Check sheet for the modelled part. Datum: model origin and axes. Units: mm. A direction names the side the tool comes from. Round coordinates to 2 decimals unless told otherwise and drop trailing zeros. Loops run counter-clockwise (first coordinate to the right, second up) from the corner with the lowest first, then second, coordinate; pieces in that order, holes last. Notation, with made-up numbers: (-19.5, -19.75) - (-9.5, -19.75) arc R24 cw to (-9.5, 14.25) - close; hole circle Ø6 at (-25, -6.5). An arc over 180 degrees is marked (long way). Answer in a Markdown table with one row per item. Add a question column.
(1) Mould release check, pull along X, two halves, no side actions. Record for faces 1 (the cylindrical face through (-0.385, -11.515, -0.022)), 2 (the flat face through (-42, 19, -2.921)), 3 (the cylindrical face through (-11.012, -49.592, 0.041)): +X half, -X half, draft (parallel to the pull), parting line (faces both ways), or undercut.
(2) Cross-section at D-D on y = 28.5. Enter the section's corners in (x, z), then the cut area to 3 significant figures.
(3) Cross-section at C-C on z = -0.25. Count the separate pieces of the cut face and the enclosed holes in it, then the cut area to 3 significant figures.
(4) Gauge pin test, flat ends, axial feed: pin 1 (4.5 mm diameter, centred on x = -6.91, y = -6.91, fed in from -Z); pin 2 (5 mm diameter, centred on x = 18.5, y = -5.5, fed in from +Z); pin 3 (3 mm diameter, centred on x = -9.779, y = 0, fed in from +Z); pin 4 (1.5 mm diameter, centred on x = 30.5, z = 1.5, fed in from -Y). Record the tip position at first contact, or that the pin passes through.
(5) Access from +Z, -Z, +X, -X, +Y, -Y to the whole of each face (thin tool, end or side, straight path). Record for faces 4 (the cylindrical face through (43.61, 13.73, 2.24)), 5 (the flat face through (10, -10, -1.588)), 6 (the cylindrical face through (0, 8, 0)).
(6) Thickness scan on line 1 along X through (y, z) = (0.5, -1.4); line 2 along Z through (x, y) = (13, -31); line 3 along X through (y, z) = (-18.5, -2.45). Record the ranges inside material, lowest first.
(7) Cross-section at A-A on x = 0. Enter the section's corners in (y, z), then the cut area to 3 significant figures.
from build123d import *

# Parameters (mm, degrees)
SKETCH1_R           = 50.8
SKETCH1_R_2         = 45.72
BOSS_EXTRUDE1_DEPTH = 2.921
SKETCH3_R           = 45.72
SKETCH3_R_2         = 6.35
SKETCH3_R_3         = 1.778
BOSS_EXTRUDE2_DEPTH = 1.5875


with BuildPart() as part:
    # Sketch1 → Boss-Extrude1 (new body, symmetric)
    with BuildSketch(Plane.XY):
        Circle(SKETCH1_R)
        Circle(SKETCH1_R_2, mode=Mode.SUBTRACT)
    extrude(amount=BOSS_EXTRUDE1_DEPTH, both=True)

    # Sketch3 → Boss-Extrude2 (add, symmetric)
    with BuildSketch(Plane.XY):
        Circle(SKETCH3_R)
        Circle(SKETCH3_R_2, mode=Mode.SUBTRACT)
        with Locations((0, 9.779)):
            Circle(SKETCH3_R_3, mode=Mode.SUBTRACT)
        with Locations((6.914797213, 6.914797213)):
            Circle(SKETCH3_R_3, mode=Mode.SUBTRACT)
        with Locations((9.779, 0)):
            Circle(SKETCH3_R_3, mode=Mode.SUBTRACT)
        with Locations((6.914797213, -6.914797213)):
            Circle(SKETCH3_R_3, mode=Mode.SUBTRACT)
        with Locations((0, -9.779)):
            Circle(SKETCH3_R_3, mode=Mode.SUBTRACT)
        with Locations((-6.914797213, -6.914797213)):
            Circle(SKETCH3_R_3, mode=Mode.SUBTRACT)
        with Locations((-9.779, 0)):
            Circle(SKETCH3_R_3, mode=Mode.SUBTRACT)
        with Locations((-6.914797213, 6.914797213)):
            Circle(SKETCH3_R_3, mode=Mode.SUBTRACT)
    extrude(amount=BOSS_EXTRUDE2_DEPTH, both=True)


solid = part.part
Answers:
| question | item | result |
|---|---|---|
| 1 | face 1 | undercut |
| 1 | face 2 | draft |
| 1 | face 3 | parting line |
| 2 | outline | (-42.05, -2.92) - (-35.75, -2.92) - (-35.75, -1.59) - (35.75, -1.59) - (35.75, -2.92) - (42.05, -2.92) - (42.05, 2.92) - (35.75, 2.92) - (35.75, 1.59) - (-35.75, 1.59) - (-35.75, 2.92) - (-42.05, 2.92) - close |
| 2 | area | 301 mm^2 |
| 3 | separate pieces | 1 |
| 3 | enclosed holes | 9 |
| 3 | area | 7,900 mm^2 |
| 4 | pin 1 | stops at z = -1.59 |
| 4 | pin 2 | stops at z = 1.59 |
| 4 | pin 3 | passes through |
| 4 | pin 4 | stops at y = -41.18 |
| 5 | face 4 | +Z |
| 5 | face 5 | -Z |
| 5 | face 6 | +Z, -Z |
| 6 | line 1 | x = -50.8 to -11.49, -8.07 to -6.33, 6.33 to 8.07, 11.49 to 50.8 |
| 6 | line 2 | z = -1.59 to 1.59 |
| 6 | line 3 | x = -47.31 to -41.81, 41.81 to 47.31 |
| 7 | outline | (-50.8, -2.92) - (-45.72, -2.92) - (-45.72, -1.59) - (-11.56, -1.59) - (-11.56, 1.59) - (-45.72, 1.59) - (-45.72, 2.92) - (-50.8, 2.92) - close; (-8, -1.59) - (-6.35, -1.59) - (-6.35, 1.59) - (-8, 1.59) - close; (6.35, -1.59) - (8, -1.59) - (8, 1.59) - (6.35, 1.59) - close; (11.56, -1.59) - (45.72, -1.59) - (45.72, -2.92) - (50.8, -2.92) - (50.8, 2.92) - (45.72, 2.92) - (45.72, 1.59) - (11.56, 1.59) - close |
| 7 | area | 287 mm^2 |
